Source: three-view drawing plus pictorial views. Frame: mm from the lowest corner of the part. Give positions to 0.01 mm unless a question says otherwise; leave off trailing zeros. Loops run counter-clockwise (first coordinate to the right, second up) from the corner with the lowest first, then second, coordinate; pieces in that order, holes last. Notation, with made-up numbers: M 77.25,-32.5 L 91.25,-32.5 A18 cw 91.25,-26.5 Z; hole C 31.25,48.5 d7. An arc over 180 degrees is marked long. Put each result on its own line as item: value. Start each with the question number.
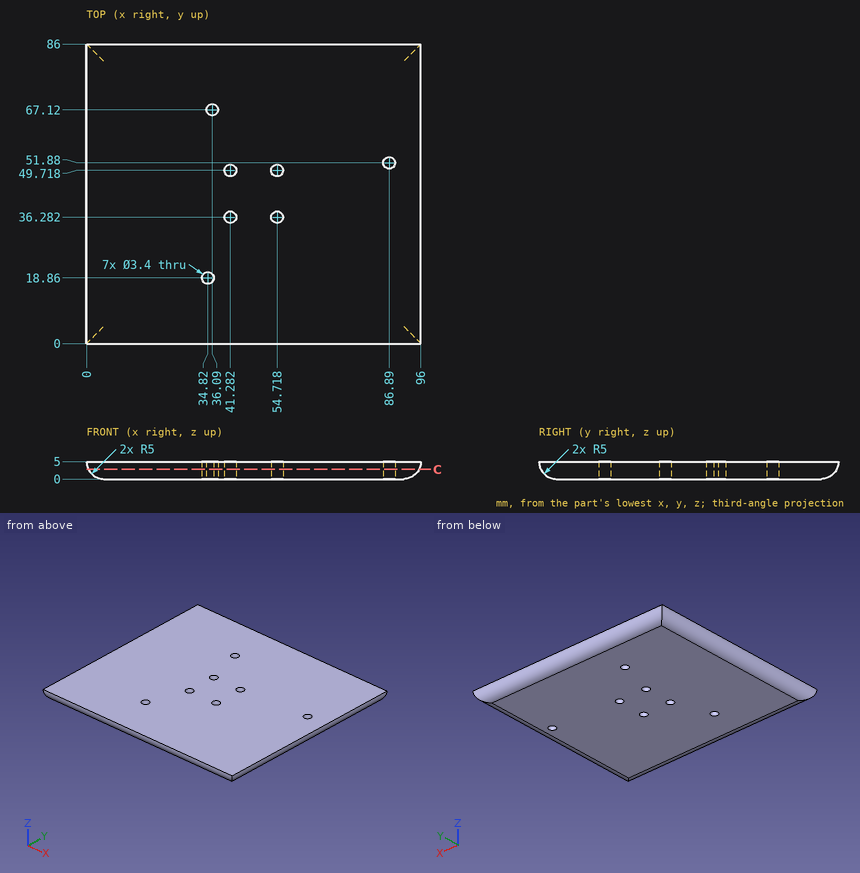
1. Ray query, line 1 (X direction, y = 50, z = 4.25) (1 decimal); line 2 (Y direction, x = 41.5, z = 1.7) (1 decimal); line 3 (Y direction, x = 40.5, z = 1.1) (1 decimal). Return the intervals inside material, ascending.
2. Section C-C, the plane z = 2.75. Output: boundary loops of the cut face in (x, y) (1 decimal), plus the area to 3 significant figures.
3. Contact query for flat-ended pins moving along their axis: pin 1 (2 mm diameter, centred on x = 17.5, z = 3.5, fed in from +Y) (1 decimal); pin 2 (2 mm diameter, centred on x = 36.09, y = 67.12, fed in from +Z). Output: stop coordinate, or through.
Results found:
1. line 1: 0.1 to 39.6, 43 to 53, 56.4 to 95.9
1. line 2: 1.2 to 34.6, 38 to 48, 51.4 to 84.8
1. line 3: 1.9 to 34.8, 37.8 to 48.2, 51.2 to 84.1
2. outline: M 0.5,0.5 L 95.5,0.5 L 95.5,85.5 L 0.5,85.5 Z; hole C 34.8,18.9 d3.4; hole C 36.1,67.1 d3.4; hole C 41.3,36.3 d3.4; hole C 41.3,49.7 d3.4; hole C 54.7,36.3 d3.4; hole C 54.7,49.7 d3.4; hole C 86.9,51.9 d3.4
2. area: 8,000 mm²
3. pin 1: y = 86
3. pin 2: through
